```python
from build123d import *

# Parameters (mm, degrees)
SKETCH_3_R        = 1
SWEEP_START       = 35
SWEEP_6_OUTLINE_R = 1
SWEEP_6_DEPTH     = 30


# Read off the part's stored shape, not the designer's step: ｽｲｰﾌﾟ6
with BuildPart() as part:
    # ｽｲｰﾌﾟ3: sweep along a path in ｽｹｯﾁ4
    with BuildLine(Plane.XY) as sweep_3_path:
        Line((0, 0), (34.999999999999936, 0))
        ThreePointArc((34.999999999999936, 0), (42.071067811865476, -2.9289321881345254), (45, -10.000000000000066))
        Line((45, -10.000000000000066), (45.000000000000014, -50))
    # ｽｹｯﾁ3 → ｽｲｰﾌﾟ3 (sweep)
    with BuildSketch(Plane(origin=(0, 0, 0), x_dir=(0, 0, -1), z_dir=(1, 0, 0))):
        Circle(SKETCH_3_R)
    sweep(path=sweep_3_path.line)

    # ｽｲｰﾌﾟ6 outline → ｽｲｰﾌﾟ6 (add)
    with BuildSketch(Plane.YZ.offset(SWEEP_START)):
        Circle(SWEEP_6_OUTLINE_R)
    extrude(amount=SWEEP_6_DEPTH)


solid = part.part
```
Source: CAD feature listing. Evaluate the final solid. Frame: model axes, mm. A direction names the side the tool comes from. Give positions to 0.01 mm unless a question says otherwise; leave off trailing zeros. Order: outer loops, then holes, each group sorted by start corner. A loop starts at its lowest first (then second) coordinate and runs counter-clockwise, first axis right, second up. Notation, with made-up numbers: (87.5, 31.5) -> (124.5, 31.5) arc R35 cw to (124.5, 69.5) -> close; hole circle Ø2 at (37, 46). An arc over 180 degrees is marked (long way). Use a Markdown table: item, result.
Q1. Section B-B (z = 0). Return the cut outline in (x, y), and give its area (3 significant figures).
A:
| item | result |
|---|---|
| outline | (0, -1) -> (35, -1) arc R9 cw to (44, -10) -> (44, -50) -> (46, -50) -> (46, -10) arc R11 ccw to (41.32, -1) -> (65, -1) -> (65, 1) -> (0, 1) -> close |
| area | 233 mm^2 |
Q2. Material intervals for line 1 (Y direction, x = 45, z = -0.15); line 2 (X direction, y = -8, z = -0.15); line 3 (Y direction, x = 46.5, z = 0.05), sorted ascending. Write a range as [from, to].
A:
| item | result |
|---|---|
| line 1 | [-50, -5.44], [-0.99, 0.99] |
| line 2 | [43.79, 45.81] |
| line 3 | [-1, 1] |
Q3. Access query for faces 1 (the face through (46, -30, 0)), 2 (the face through (0, 0, 0)). Directions: +Z, -Z, +X, -X, +Y, -Y. A direction counts if a zero-diameter tool reaches every point of the face in a straight line with its end or side. Return the directions, or none.
A:
| item | result |
|---|---|
| face 1 | -Y |
| face 2 | +Z, -Z, -X, +Y, -Y |
Q4. Section A-A (x = 29). Return the cut outline in (y, z).
A:
| item | result |
|---|---|
| outline | circle Ø2 at (0, 0) |
Q5. Section C-C (y = -22.5). Return the cut outline in (x, z).
A:
| item | result |
|---|---|
| outline | circle Ø2 at (45, 0) |
